Read the model definition and answer for the solid it produces. Units are mm, in the model's axes. A direction names the side the tool comes from. Give positions to 0.01 mm unless a question says otherwise; leave off trailing zeros. Loops run counter-clockwise (first coordinate to the right, second up) from the corner with the lowest first, then second, coordinate; pieces in that order, holes last. Notation, with made-up numbers: (-6.75, 45.25) - (41.25, 45.25) arc R21 cw to (41.25, 77.25) - close; hole circle Ø7 at (49.25, 48). An arc over 180 degrees is marked (long way). Write item = value, one per line.
```python
from build123d import *

# Parameters (mm, degrees)
SKETCH2_R           = 8.5
SKETCH2_R_2         = 3.3
BOSS_EXTRUDE1_DEPTH = 2
SKETCH2_4_R         = 8.5
BOSS_EXTRUDE2_DEPTH = 5.5
SKETCH3_R           = 8.5
SKETCH3_R_2         = 3.3
BOSS_EXTRUDE3_DEPTH = 9


with BuildPart() as part:
    # Sketch2 → Boss-Extrude1 (new body)
    with BuildSketch(Plane(origin=(0, 0, 0), x_dir=(1, 0, 0), z_dir=(0, 1, 0))):
        with Locations(Location((0, 0, 0), (0, 0, 270))):
            Circle(SKETCH2_R)
        Polygon((-3.204293994, 5.55), (-6.408587988, 0), (-3.204293994, -5.55), (3.204293994, -5.55), (6.408587988, 0), (3.204293994, 5.55), align=None, mode=Mode.SUBTRACT)
        Polygon((3.204293994, 5.55), (-3.204293994, 5.55), (-6.408587988, 0), (-3.204293994, -5.55), (3.204293994, -5.55), (6.408587988, 0), align=None)
        with Locations(Location((0, 0, 0), (0, 0, 270))):
            Circle(SKETCH2_R_2, mode=Mode.SUBTRACT)
    extrude(amount=BOSS_EXTRUDE1_DEPTH)

    # Sketch2_4 → Boss-Extrude2 (add)
    with BuildSketch(Plane(origin=(0, 0, 0), x_dir=(1, 0, 0), z_dir=(0, 1, 0))):
        with Locations(Location((0, 0, 0), (0, 0, 270))):
            Circle(SKETCH2_4_R)
        Polygon((-3.204293994, 5.55), (-6.408587988, 0), (-3.204293994, -5.55), (3.204293994, -5.55), (6.408587988, 0), (3.204293994, 5.55), align=None, mode=Mode.SUBTRACT)
    extrude(amount=-BOSS_EXTRUDE2_DEPTH)

    # Sketch3 → Boss-Extrude3 (add)
    with BuildSketch(Plane(origin=(0, 2, 0), x_dir=(1, 0, 0), z_dir=(0, 1, 0))):
        with Locations(Location((0, 0, 0), (0, 0, 270))):
            Circle(SKETCH3_R)
        with Locations(Location((0, 0, 0), (0, 0, 270))):
            Circle(SKETCH3_R_2, mode=Mode.SUBTRACT)
    extrude(amount=BOSS_EXTRUDE3_DEPTH)


solid = part.part
```
1) Each of these flat-tipped pins is pushed along its axis until it touches: P1, Ø1, axis at x = -1, y = 2.5, coming from the -Z side; P2, Ø1.5, axis at x = 4.5, y = -3, coming from the +Z side; P3, Ø1, axis at x = 2.5, z = -2, coming from the -Y side. Where does it stop, or does it pass through?
Output:
P1 = -8.49
P2 = 7.63
P3 = 0
2) A cutting plane is placed at A-A on x = 0. Determine the outline of the cut face in (y, z).
Output:
outline = (-5.5, -8.5) - (11, -8.5) - (11, -3.3) - (0, -3.3) - (0, -5.55) - (-5.5, -5.55) - close; (-5.5, 5.55) - (0, 5.55) - (0, 3.3) - (11, 3.3) - (11, 8.5) - (-5.5, 8.5) - close
3) A cutting plane is placed at C-C on y = 5.5. Determine the outline of the cut face in (x, z), then the cut area to 3 significant figures.
Output:
outline = circle Ø17 at (0, 0); hole circle Ø6.6 at (0, 0)
area = 193 mm²
4) Find the intervals of material crossed by probe 1 along X at (y, z) = (5.5, 0); probe 2 along Y at (x, z) = (3.75, 2); probe 3 along Z at (x, y) = (-1.5, -3.75), in increasing order.
Output:
probe_1 = -8.5 to -3.3, 3.3 to 8.5
probe_2 = 0 to 11
probe_3 = -8.37 to -5.55, 5.55 to 8.37
5) A tool of negligible diameter and unlimited length cuts with its end or side. For faces 4 (the face through (-6, -5.5, -2)), 5 (the face through (-4.784, -2.712, -2.814)), from which of +Z, -Z, +X, -X, +Y, -Y can it reach the whole face along a straight path? Write none if from no direction.
Output:
face_4 = +Z, -Z, +X, -X, -Y
face_5 = -Y
6) A cutting plane is placed at D-D on z = -4. Determine the outline of the cut face in (x, y), then the cut area to 3 significant figures.
Output:
outline = (-7.5, -5.5) - (-4.1, -5.5) - (-4.1, 0) - (4.1, 0) - (4.1, -5.5) - (7.5, -5.5) - (7.5, 11) - (-7.5, 11) - close
area = 202 mm²
7) A cutting plane is placed at B-B on z = 2. Determine the outline of the cut face in (x, y), then the cut area to 3 significant figures.
Output:
outline = (-8.26, -5.5) - (-5.25, -5.5) - (-5.25, 0) - (-2.62, 0) - (-2.62, 11) - (-8.26, 11) - close; (2.62, 0) - (5.25, 0) - (5.25, -5.5) - (8.26, -5.5) - (8.26, 11) - (2.62, 11) - close
area = 157 mm²
8) The mould has two halves that part along Z. Classify faces 1 (the face through (-4.829, -2.712, 2.736)), 2 (the face through (8.428, 2.634, -1.107)), 3 (the face through (0, 11, 4)): pulls with the +Z half, pulls with the -Z half, needs draft (parallel to the pull), parting line crosses it, or undercut.
Output:
face_1 = undercut
face_2 = parting line crosses it
face_3 = needs draft
